Autodesk Inventor part; units mm, degrees
ref_plane "YZ Plane" through (0, 0, 0) normal (1, 0, 0) x (0, 1, 0)
ref_plane "XZ Plane" through (0, 0, 0) normal (0, 1, 0) x (-1, 0, 0)
ref_plane "XY Plane" through (0, 0, 0) normal (0, 0, 1) x (1, 0, 0)
sketch "Sketch1" plane through (0, 0, 0) normal (0, 0, 1) x (1, 0, 0)
  arc A0 (28.575, 0) -> (-28.575, 0) centre (0, 0) ccw
  circle A1 centre (0, 0) radius 7
  line L0 (-19, -50.8) -> (19, -50.8)
  line L1 (28.575, -25.4) -> (28.575, 0)
  line L2 (-28.575, 0) -> (-28.575, -25.4)
  line L3 (0, -66.675) -> (0, 44.45)
  circle A2 centre (-12.7, -38.1) radius 2.5781
  circle A3 centre (12.7, -38.1) radius 2.5781
  line L4 (-19, -50.8) -> (-50.8, -50.8)
  line L5 (-50.8, -50.8) -> (-50.8, -25.4)
  line L6 (50.8, -25.4) -> (50.8, -50.8)
  line L7 (50.8, -50.8) -> (-50.8, -50.8)
  line L8 (-50.8, -25.4) -> (-28.575, -25.4)
  line L9 (28.575, -25.4) -> (50.8, -25.4)
  circle A4 centre (-38.1, -38.1) radius 2.5781
  circle A5 centre (38.1, -38.1) radius 2.5781
  dimension "d1" = 14
  dimension "d10" = 5.1562
  dimension "d11" = 5.1562
  dimension "d12" = 12.7
  dimension "d13" = 12.7
  dimension "d14" = 12.7
  dimension "d15" = 12.7
  dimension "d16" = 50.8
  dimension "d17" = 25.4
  dimension "d18" = 101.6
  dimension "d19" = 50.8
  dimension "d20" = 25.4
  dimension "d21" = 25.4
  dimension "d25" = 28.575
  dimension "d26" = 25.4
extrude "Extrusion1" add sketch "Sketch1" along normal blind 3.302 contours L1 L9 L6 L7 L0 L3 A1 A0 | L3 A1 L0 L4 L5 L8 L2 A0
fillet "Fillet1" radius 3.175 6 edges at (28.575, -25.4, 1.651) (-28.575, -25.4, 1.651) (-50.8, -25.4, 1.651) (-50.8, -50.8, 1.651) (50.8, -25.4, 1.651) (50.8, -50.8, 1.651)
sketch "Sketch2" plane through (0, 0, 3.302) normal (0, 0, 1) x (1, 0, 0)
  circle A0 centre (0, 0) radius 12
  circle A1 centre (0, 0) radius 20.955
  circle A2 centre (0, 0) radius 7
  line L0 (0, 0) -> (14.8174, 14.8174)
  line L1 (0, 0) -> (12, 0) construction
  line L2 (0, 0) -> (0, 12) construction
  dimension "d28" = 41.91
  dimension "d27" = 24
  dimension "d29" = 45
hole "Hole1" at (14.8174, 14.8174, 3.302) direction (0, 0, -1) diameter 5.1054 depth 16.256 tip angle 118
pattern_circular "Circular Pattern1" count 4 over 360 about axis through (0, 0, 0) along (0, 0, 1) of "Hole1"
hole "Hole2" at (0, 12, 3.302) direction (0, 0, -1) diameter 4.4958 depth 16.256 tip angle 118
pattern_circular "Circular Pattern2" count 4 over 360 about axis through (0, 0, 0) along (0, 0, 1) of "Hole2"
equation "\"d19\" = 0.5 * d18"
properties part number "ArmPlateBase V2"
Verification items for the finished model (mm, model axes). A direction names the side the tool comes from. Coordinates: 2 decimals unless noted, no trailing zeros. Loops run counter-clockwise (first coordinate to the right, second up) from the corner with the lowest first, then second, coordinate; pieces in that order, holes last. Notation, with made-up numbers: M 73.25,-10.5 L 81.25,-10.5 A11 ccw 81.25,7.5 Z; hole C 56.5,24.5 d11. An arc over 180 degrees is marked long. One line per item, written item: value.
1. Section check C-C on z = 2.5. Give the number of separate pieces and of enclosed holes in the cut face, plus the area to 3 significant figures.
Answers follow:
separate pieces: 1
enclosed holes: 13
area: 4,930 mm^2
2. Section check B-B on x = -38.1. Record the cut outline in (y, z), plus the area to 3 significant figures.
Answers follow:
outline: M -50.8,0 L -40.68,0 L -40.68,3.3 L -50.8,3.3 Z; M -35.52,0 L -25.4,0 L -25.4,3.3 L -35.52,3.3 Z
area: 66.8 mm^2
3. Section check A-A on x = 0. Record the cut outline in (y, z) (3 decimals).
Answers follow:
outline: M -50.8,0 L -14.248,0 L -14.248,3.302 L -50.8,3.302 Z; M -9.752,0 L -7,0 L -7,3.302 L -9.752,3.302 Z; M 7,0 L 9.752,0 L 9.752,3.302 L 7,3.302 Z; M 14.248,0 L 28.575,0 L 28.575,3.302 L 14.248,3.302 Z
4. Section check D-D on y = -21. Record the cut outline in (x, z) (3 decimals).
Answers follow:
outline: M -28.575,0 L 28.575,0 L 28.575,3.302 L -28.575,3.302 Z
5. Mould release check, pull along Y, two halves, no side actions. Record for faces 1 (the cylindrical face through (-35.64, -38.87, 1.63)), 2 (the cylindrical face through (49.89, -26.35, 1.67)), 3 (the flat face through (28.575, -11, 2)): pulls with the +Y half, pulls with the -Y half, needs draft (parallel to the pull), parting line crosses it, or undercut.
Answers follow:
face 1: undercut
face 2: pulls with the +Y half
face 3: needs draft
6. Set-up check for faces 4 (the flat face through (-40, -25.4, 2)), 5 (the flat face through (40, -25.4, 2)), 6 (the flat face through (50.8, -38, 2)): record each of +Z, -Z, +X, -X, +Y, -Y from which the full face is reachable in a straight line by a thin tool's end or side.
Answers follow:
face 4: +Z, -Z, -X, +Y
face 5: +Z, -Z, +X, +Y
face 6: +Z, -Z, +X, +Y, -Y
7. Gauge pin test, flat end, axial feed: P1, Ø1.7, axis at y = -15, z = 2, coming from the -X side (3 decimals). Record the tip position at first contact, or that the pin passes through.
Answers follow:
P1: x = -28.575
8. Material ranges on line 1 along X through (y, z) = (-12, 1.55) (3 decimals); line 2 along Y through (x, z) = (-38.1, 2.2); line 3 along X through (y, z) = (-13, 0.4) (3 decimals), recorded low to high. Write a range as from..to.
Answers follow:
line 1: -28.575..-2.248, 2.248..28.575
line 2: -50.8..-40.68, -35.52..-25.4
line 3: -28.575..-16.61, -13.025..-2.013, 2.013..13.025, 16.61..28.575
